Here's how the part is built. I have some questions about the finished solid (model axes, mm). Face numbers are marked on the shaded views. A direction names the side the tool comes from. Round coordinates to 2 decimals unless told otherwise and drop trailing zeros. Loops run counter-clockwise (first coordinate to the right, second up) from the corner with the lowest first, then second, coordinate; pieces in that order, holes last. Notation, with made-up numbers: M 48,43.5 L 80,43.5 A15 cw 80,70.5 Z; hole C -9,59 d6. An arc over 180 degrees is marked long. Use a Markdown table: item, result.
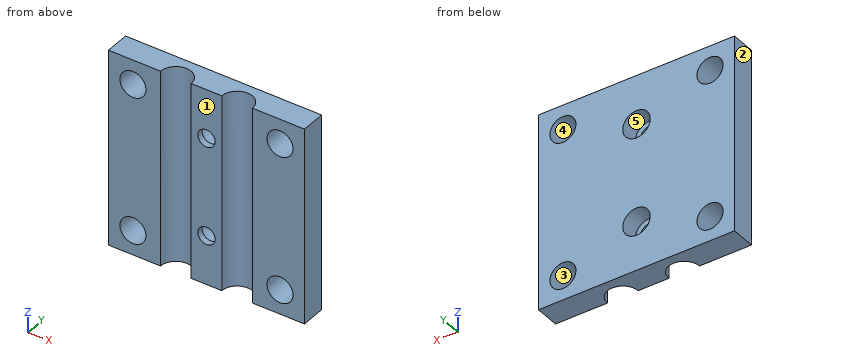
```python
from build123d import *

# Parameters (mm, degrees)
SKETCH1_W               = 50.8
SKETCH1_H               = 50.8
BOSS_EXTRUDE1_DEPTH     = 6.35
SKETCH2_R               = 3.96875
CUT_EXTRUDE1_DEPTH      = 58.15
F_1_4_CLEARANCE_HOLE1_D = 6.7564
F_8_CLEARANCE_HOLE1_D   = 4.4958
SKETCH10_R              = 3.556
CUT_EXTRUDE2_DEPTH      = 4.7625


with BuildPart() as part:
    # Sketch1 → Boss-Extrude1 (new body)
    with BuildSketch(Plane(origin=(0, 0, 0), x_dir=(1, 0, 0), z_dir=(0, 1, 0))):
        Rectangle(SKETCH1_W, SKETCH1_H)
    extrude(amount=BOSS_EXTRUDE1_DEPTH)

    # Sketch2 → Cut-Extrude1 (cut, through all)
    with BuildSketch(Plane.XY.offset(25.4)):
        with Locations((-7.9375, 0)):
            Circle(SKETCH2_R)
        with Locations((7.9375, 0)):
            Circle(SKETCH2_R)
    extrude(amount=-CUT_EXTRUDE1_DEPTH, mode=Mode.SUBTRACT)

    # 1/4 Clearance Hole1 (through all)
    with Locations(Plane(origin=(0, 6.35, 0), x_dir=(1, 0, 0), z_dir=(0, 1, 0))):
        with Locations((-19.05, -19.05), (-19.05, 19.05), (19.05, 19.05), (19.05, -19.05)):
            Hole(F_1_4_CLEARANCE_HOLE1_D / 2)

    # #8 Clearance Hole1 (through all)
    with Locations(Plane(origin=(0, 6.35, 0), x_dir=(1, 0, 0), z_dir=(0, 1, 0))):
        with Locations((0, 12.7), (0, -12.7)):
            Hole(F_8_CLEARANCE_HOLE1_D / 2)

    # Sketch10 → Cut-Extrude2 (cut)
    with BuildSketch(Plane(origin=(0, 6.35, 0), x_dir=(1, 0, 0), z_dir=(0, 1, 0))):
        with Locations(Location((0, 12.7, 0), (0, 0, 270))):
            Circle(SKETCH10_R)
        with Locations(Location((0, -12.7, 0), (0, 0, 270))):
            Circle(SKETCH10_R)
    extrude(amount=-CUT_EXTRUDE2_DEPTH, mode=Mode.SUBTRACT)


solid = part.part
```
Q1. Imagine slicing it at D-D, the plane x = 0. Please give me the cut outline in (y, z).
Return value:
| item | result |
|---|---|
| outline | M 0,-25.4 L 6.35,-25.4 L 6.35,-16.26 L 1.59,-16.26 L 1.59,-14.95 L 0,-14.95 Z; M 0,-10.45 L 1.59,-10.45 L 1.59,-9.14 L 6.35,-9.14 L 6.35,9.14 L 1.59,9.14 L 1.59,10.45 L 0,10.45 Z; M 0,14.95 L 1.59,14.95 L 1.59,16.26 L 6.35,16.26 L 6.35,25.4 L 0,25.4 Z |
Q2. For the marked faces 4 and 5, which set-ups out of +Z, -Z, +X, -X, +Y, -Y let a thin tool reach every point of the face, with its end or its side?
Return value:
| item | result |
|---|---|
| face 4 | +Y, -Y |
| face 5 | +Y |
Q3. Imagine slicing it at B-B, the plane z = 12.7. Please give me the cut outline in (x, y).
Return value:
| item | result |
|---|---|
| outline | M -25.4,0 L -11.91,0 A3.97 cw -3.97,0 L -2.25,0 L -2.25,1.59 L -3.56,1.59 L -3.56,6.35 L -25.4,6.35 Z; M 2.25,0 L 3.97,0 A3.97 cw 11.91,0 L 25.4,0 L 25.4,6.35 L 3.56,6.35 L 3.56,1.59 L 2.25,1.59 Z |
Q4. Will these pins go through, and if not, where does the flat tip stop? P1, Ø5.5, axis at x = -19.05, z = 19.05, coming from the +Y side (1 decimal); P2, Ø7, axis at x = 0, z = -12.7, coming from the +Y side; P3, Ø4, axis at x = -6.5, z = 18, coming from the -Y side.
Return value:
| item | result |
|---|---|
| P1 | passes through |
| P2 | stops at y = 1.59 |
| P3 | stops at y = 1.98 |
Q5. Imagine slicing it at A-A, the plane x = 19.05. Please give me the cut outline in (y, z), then the cut area to 3 significant figures.
Return value:
| item | result |
|---|---|
| outline | M 0,-25.4 L 6.35,-25.4 L 6.35,-22.43 L 0,-22.43 Z; M 0,-15.67 L 6.35,-15.67 L 6.35,15.67 L 0,15.67 Z; M 0,22.43 L 6.35,22.43 L 6.35,25.4 L 0,25.4 Z |
| area | 237 mm^2 |
Q6. I need wall thicknesses on line 1 (Z direction, x = -19.05, y = 2.25); line 2 (Z direction, x = 0, y = 0.55); line 3 (X direction, y = 4.55, z = 12.7). Which ranges of each line are inside material? Lowest first, please. Write a range as from..to.
Return value:
| item | result |
|---|---|
| line 1 | z = -25.4..-22.43, -15.67..15.67, 22.43..25.4 |
| line 2 | z = -25.4..-14.95, -10.45..10.45, 14.95..25.4 |
| line 3 | x = -25.4..-3.56, 3.56..25.4 |
Q7. We'd pull the mould along X, two halves only. Please class the marked faces 1, 2 and 3: pulls with the +X half, pulls with the -X half, needs draft (parallel to the pull), parting line crosses it, or undercut.
Return value:
| item | result |
|---|---|
| face 1 | needs draft |
| face 2 | pulls with the -X half |
| face 3 | undercut |
Q8. Imagine slicing it at C-C, the plane z = -19.05. Please give me the cut outline in (x, y), then the cut area to 3 significant figures.
Return value:
| item | result |
|---|---|
| outline | M -25.4,0 L -22.43,0 L -22.43,6.35 L -25.4,6.35 Z; M -15.67,0 L -11.91,0 A3.97 cw -3.97,0 L 3.97,0 A3.97 cw 11.91,0 L 15.67,0 L 15.67,6.35 L -15.67,6.35 Z; M 22.43,0 L 25.4,0 L 25.4,6.35 L 22.43,6.35 Z |
| area | 187 mm^2 |
